from build123d import *

# Parameters (mm, degrees)
F2_R = 5.08
F3_T = -2.54
F5_D = 25.4


# Not quite as in the source:
# - a shell that OpenCascade refuses in one call is made with other operations: the cavity is built on its own and cut out


with BuildPart() as f1:
    # F0 (on Front) → F1 (revolve)
    with BuildSketch(Plane.XZ):
        Polygon((0, 50.8), (0, 0), (50.8, 50.8), align=None)
    revolve(axis=Axis((0, 0, 25.4), (0, 0, 1)))

    # F2
    f2_edges = [f1.edges().sort_by_distance(p)[0] for p in [
        (-50.8, 0, 50.8),
    ]]
    fillet(f2_edges, radius=F2_R)

    # F3: a shell. OpenCascade refuses it in one call, so the cavity is built on its own and cut out:
    # the body offset inwards by the wall thickness, plus a prism from it out through each open face.
    f3_core = offset(f1.part, amount=F3_T, mode=Mode.PRIVATE)
    f3_exits = [f3_core.faces().sort_by_distance(p)[0] for p in [
        (0, 0, 48.26),
    ]]
    add(f3_core, mode=Mode.SUBTRACT)
    extrude(f3_exits, amount=-F3_T, mode=Mode.SUBTRACT)

    # F5 (through all)
    with Locations(Plane(origin=(0, 0, 0), x_dir=(1, 0, 0), z_dir=(0, 0, -1))):
        with Locations((0, 0)):
            Hole(F5_D / 2)


solid = f1.part
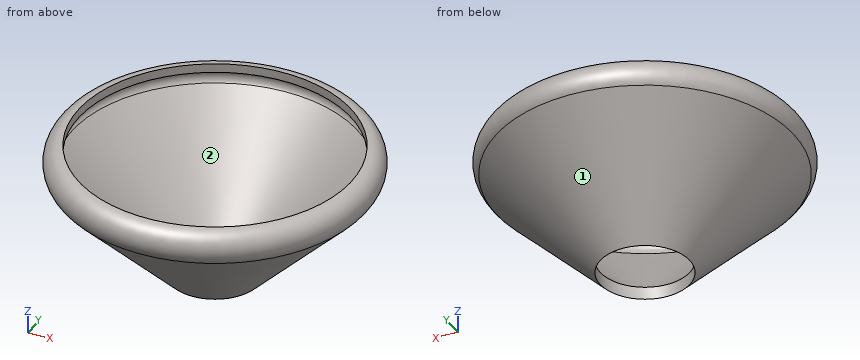
Source: CAD feature listing. Evaluate the final solid. Frame: model axes, mm. Face numbers are marked on the shaded views. Give positions to 0.01 mm unless a question says otherwise; leave off trailing zeros. Write each loop counter-clockwise with the first axis right and the second up, starting at its lowest first coordinate (ties: lowest second). Pieces come first, ordered by that corner, then holes. Notation, with made-up numbers: M -34,49 L 12,49 A17 ccw 12,57 Z; hole C 26.25,-25.75 d10. An arc over 180 degrees is marked long. Return JSON: item names as keys, results as strings. Group by question number.
1) Draft query along Y for the marked faces 1 and 2. Return one class per face: released by +Y, released by -Y, zero draft, split by the parting line, or undercut.
2) First-contact query: pin 1 Ø3 at (y, z) = (-8.5, 31.5) entering from +X; pin 2 Ø3 at (y, z) = (5, 39.5) entering from +X; pin 3 Ø5 at (x, y) = (-0.5, 23.5) entering from +Z. Flat tips, straight axial feed; report the tip coordinate or a pass-through.
3) Ray query, L1, parallel to X at y = -5, z = 32.5; L2, parallel to Y at x = -26.5, z = 38.5; L3, parallel to Y at x = -9, z = 15. Return the intervals inside material, ascending.
4) Cut plane D-D, the plane z = 19.5. Output: boundary loops of the cut face in (x, y), then the cut area to 3 significant figures.
5) Cut plane A-A, the plane y = 0. Output: boundary loops of the cut face in (x, z), then the cut area to 3 significant figures.
6) Cut plane C-C, the plane z = 40. Output: boundary loops of the cut face in (x, y).
Data:
{
 "1": {"face 1": "split by the parting line", "face 2": "undercut"},
 "2": {"pin 1": "stops at x = 31.94", "pin 2": "stops at x = 40.7", "pin 3": "stops at z = 29.6"},
 "3": {"L1": "x = -32.11 to -28.47, 28.47 to 32.11", "L2": "y = -27.93 to -22.72, 22.72 to 27.93", "L3": "y = -12 to -8.96, 8.96 to 12"},
 "4": {"outline": "C 0,0 d39; hole C 0,0 d31.82", "area": "400 mm²"},
 "5": {"outline": "M -42.13,42.13 L -12.7,12.7 L -12.7,16.29 L -40.33,43.92 A2.54 cw -38.54,48.26 L -38.54,50.8 A5.08 ccw Z; M 12.7,12.7 L 42.13,42.13 A5.08 ccw 38.54,50.8 L 38.54,48.26 A2.54 cw 40.33,43.92 L 12.7,16.29 Z", "area": "251 mm²"},
 "6": {"outline": "C 0,0 d80; hole C 0,0 d72.82"}
}
